Build history of the part. All positions in model axes, mm. Face numbers are marked on the shaded views. Give positions to 0.01 mm unless a question says otherwise; leave off trailing zeros. Order: outer loops, then holes, each group sorted by start corner. A loop starts at its lowest first (then second) coordinate and runs counter-clockwise, first axis right, second up. Notation, with made-up numbers: (85, 56) -> (99, 56) arc R27 cw to (99, 86) -> close; hole circle Ø7 at (85, 88). An arc over 180 degrees is marked (long way). Use a Markdown table: item, result. Add a question column.
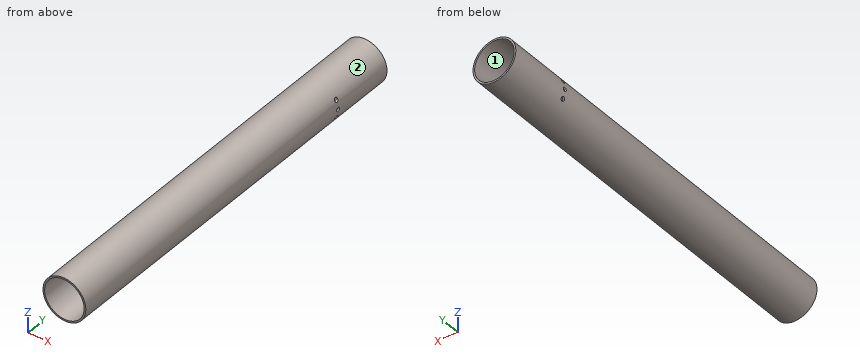
```python
from build123d import *

# Parameters (mm, degrees)
SKETCH1_R               = 55
SKETCH1_R_2             = 48.6
BOSS_EXTRUDE1_DEPTH     = 500
CUT_EXTRUDE1_DEPTH      = 507.013833803
CUT_EXTRUDE1_DEPTH_BACK = 507.013833803
SKETCH3_R               = 5
CUT_EXTRUDE2_DEPTH      = 1004.020438586
CUT_EXTRUDE2_DEPTH_BACK = 1004.020438586
SKETCH4_R               = 50.8


with BuildPart() as part:
    # Sketch1 → Boss-Extrude1 (new, symmetric)
    with BuildSketch(Plane(origin=(0, 0, 0), x_dir=(1, 0, 0), z_dir=(0, 1, 0))):
        with Locations(Location((0, 0, 0), (0, 0, 270))):
            Circle(SKETCH1_R)
        with Locations(Location((0, 0, 0), (0, 0, 270))):
            Circle(SKETCH1_R_2, mode=Mode.SUBTRACT)
    extrude(amount=BOSS_EXTRUDE1_DEPTH, both=True)

    # Sketch3 → Cut-Extrude1 (cut, two sides: drawn at the far end of the back side and taken through both)
    with BuildSketch(Plane(origin=(0, 0, 0), x_dir=(0, 0, -1), z_dir=(1, 0, 0)).offset(-CUT_EXTRUDE1_DEPTH_BACK)):
        with Locations((0, 337.5)):
            Circle(SKETCH3_R)
        with Locations((22.5, 337.5)):
            Circle(SKETCH3_R)
        with Locations((-22.5, 337.5)):
            Circle(SKETCH3_R)
    extrude(amount=CUT_EXTRUDE1_DEPTH + CUT_EXTRUDE1_DEPTH_BACK, mode=Mode.SUBTRACT)

    # Sketch4 → Cut-Extrude2 (cut, two sides: drawn at the far end of the back side and taken through both)
    with BuildSketch(Plane(origin=(0, 500, 0), x_dir=(1, 0, 0), z_dir=(0, 1, 0)).offset(-CUT_EXTRUDE2_DEPTH_BACK)):
        with Locations(Location((0, 0, 0), (0, 0, 270))):
            Circle(SKETCH4_R)
    extrude(amount=CUT_EXTRUDE2_DEPTH + CUT_EXTRUDE2_DEPTH_BACK, mode=Mode.SUBTRACT)


solid = part.part
```
(1) Pin check, flat tips, straight feed: pin 1 Ø6 at (y, z) = (337.5, 0) entering from +X; pin 2 Ø16 at (y, z) = (337.5, 22.5) entering from -X; pin 3 Ø3 at (x, y) = (-32, 399) entering from -Z; pin 4 Ø3 at (y, z) = (345, -10) entering from -X. Stop position of each tip, or through.
(2) Mould opens along Z. For the marked faces 1 and 2 say: released by +Z, released by -Z, zero draft, split by the parting line, or undercut.
(3) Band-saw the part on B-B on y = 257. Give the cut face in (x, z), plus the area to 3 significant figures.
(4) Wall check: probe 1 along Y at (x, z) = (52.8, 0); probe 2 along Z at (x, y) = (-51, 337); probe 3 along X at (y, z) = (250, 0). Give the ranges that are in metal, low to high.
(5) Band-saw the part on A-A on x = 0. Give the cut face in (y, z).
Response:
| question | item | result |
|---|---|---|
| 1 | pin 1 | passes through |
| 1 | pin 2 | stops at x = -53.05 |
| 1 | pin 3 | stops at z = -45.77 |
| 1 | pin 4 | stops at x = -54.34 |
| 2 | face 1 | undercut |
| 2 | face 2 | split by the parting line |
| 3 | outline | circle Ø110 at (0, 0); hole circle Ø101.6 at (0, 0) |
| 3 | area | 1,400 mm² |
| 4 | probe 1 | y = -500 to 332.5, 342.5 to 500 |
| 4 | probe 2 | z = -17.53 to -4.97, 4.97 to 17.53 |
| 4 | probe 3 | x = -55 to -50.8, 50.8 to 55 |
| 5 | outline | (-500, -55) -> (500, -55) -> (500, -50.8) -> (-500, -50.8) -> close; (-500, 50.8) -> (500, 50.8) -> (500, 55) -> (-500, 55) -> close |
